from build123d import *

# Parameters (mm, degrees)
BOSS_EXTRUDE1_DEPTH  = 5
M3_CLEARANCE_HOLE1_D = 3.4


with BuildPart() as part:
    # Sketch1 → Boss-Extrude1 (new, symmetric)
    with BuildSketch(Plane.XY):
        Polygon((0, 0), (0, 4.45), (5.5, 4.45), (5.5, 7.45), (-3, 7.45), (-3, 3), (-13, 3), (-13, 0), (-3, 0), align=None)
    extrude(amount=BOSS_EXTRUDE1_DEPTH, both=True)

    # M3 Clearance Hole1 (through all)
    with Locations(Plane(origin=(0, 3, 0), x_dir=(1, 0, 0), z_dir=(0, 1, 0))):
        with Locations((-8, 0)):
            Hole(M3_CLEARANCE_HOLE1_D / 2)


solid = part.part
The listing builds one solid part. Answer for the finished solid, in the listing's coordinates (mm). A direction names the side the tool comes from. Coordinates: 2 decimals unless noted, no trailing zeros. Write each loop counter-clockwise with the first axis right and the second up, starting at its lowest first coordinate (ties: lowest second). Pieces come first, ordered by that corner, then holes. Notation, with made-up numbers: (-34, 64) - (-5, 64) arc R29 cw to (-5, 94) - close; hole circle Ø2 at (57.25, 76). An arc over 180 degrees is marked (long way). Answer as CSV lines item,"result".
1. Find section B-B (z = 0). Give the vertices of the cut face in (x, y).
Computed values:
outline,"(-13, 0) - (-9.7, 0) - (-9.7, 3) - (-13, 3) - close; (-6.3, 0) - (0, 0) - (0, 4.45) - (5.5, 4.45) - (5.5, 7.45) - (-3, 7.45) - (-3, 3) - (-6.3, 3) - close"
2. Given P1, Ø1, axis at x = -4, z = -0.5, coming from the +Y side; P2, Ø1.5, axis at x = -10.5, z = 0.5, coming from the -Y side; P3, Ø2, axis at y = 2.5, z = -2, coming from the +X side; P4, Ø2, axis at y = 5.5, z = 0, coming from the -X side, each flat-ended and moving along its own axis, determine where each tip first touches the part or whether it passes through.
Computed values:
P1,"stops at y = 3"
P2,"stops at y = 0"
P3,"stops at x = 0"
P4,"stops at x = -3"
3. Find section C-C (z = -2.5). Give the vertices of the cut face in (x, y), plus the area to 4 significant figures.
Computed values:
outline,"(-13, 0) - (0, 0) - (0, 4.45) - (5.5, 4.45) - (5.5, 7.45) - (-3, 7.45) - (-3, 3) - (-13, 3) - close"
area,"68.85 mm²"
4. Determine the mould class of faces 1 (the flat face through (-4, 2, -5)), 2 (the flat face through (3, 4.45, 0)), 3 (the cylindrical face through (-6.65, 1.48, 1.03)) for opening direction Z: +Z half, -Z half, draft (parallel to the pull), parting line (faces both ways), or undercut.
Computed values:
face 1,"-Z half"
face 2,"draft"
face 3,"undercut"
5. Find section A-A (x = -8). Give the vertices of the cut face in (y, z).
Computed values:
outline,"(0, -5) - (3, -5) - (3, -1.7) - (0, -1.7) - close; (0, 1.7) - (3, 1.7) - (3, 5) - (0, 5) - close"
6. Find section D-D (y = 5.75). Give the vertices of the cut face in (x, z).
Computed values:
outline,"(-3, -5) - (5.5, -5) - (5.5, 5) - (-3, 5) - close"
7. Straight lines are drawn through the part: line 1 (Z direction, x = -8, y = 1.1); line 2 (Y direction, x = -6.5, z = 4.5); line 3 (X direction, y = 2.75, z = -3). For each, find the intervals that lie inside material, in ascending order. Write a range as [from, to].
Computed values:
line 1,"z = [-5, -1.7], [1.7, 5]"
line 2,"y = [0, 3]"
line 3,"x = [-13, 0]"
8. A tool of negligible diameter and unlimited length cuts with its end or side. For faces 4 (the flat face through (0, 2, 0)), 5 (the flat face through (-5, 0, 0)), 6 (the flat face through (-3, 5, 0)), from which of +Z, -Z, +X, -X, +Y, -Y can it reach the whole face along a straight path? Write none if from no direction.
Computed values:
face 4,"+Z, -Z, +X, -Y"
face 5,"+Z, -Z, +X, -X, -Y"
face 6,"+Z, -Z, -X, +Y"
